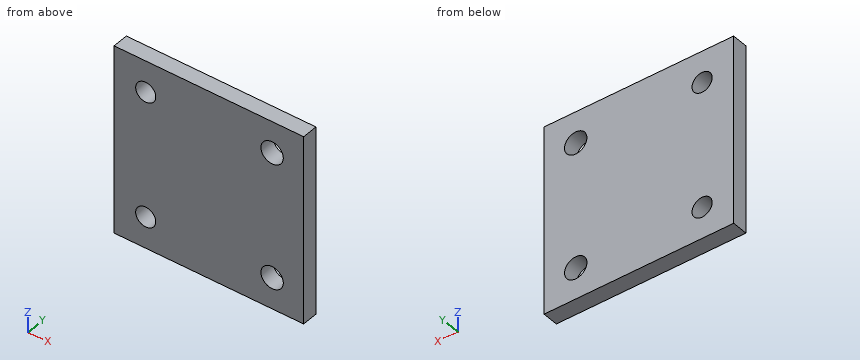
from build123d import *

# Parameters (mm, degrees)
SKETCH1_W              = 38.1
SKETCH1_H              = 38.1
BOSS_EXTRUDE1_DEPTH    = 1.5875
F_10_32_TAPPED_HOLE1_D = 4.0386
F_8_CLEARANCE_HOLE1_D  = 4.4958


with BuildPart() as part:
    # Sketch1 → Boss-Extrude1 (new, symmetric)
    with BuildSketch(Plane(origin=(0, 0, 0), x_dir=(1, 0, 0), z_dir=(0, 1, 0))):
        Rectangle(SKETCH1_W, SKETCH1_H)
    extrude(amount=BOSS_EXTRUDE1_DEPTH, both=True)

    # #10-32 Tapped Hole1 (through all)
    with Locations(Plane(origin=(0, 1.5875, 0), x_dir=(1, 0, 0), z_dir=(0, 1, 0))):
        with Locations((-12.7, 12.7), (-12.7, -12.7)):
            Hole(F_10_32_TAPPED_HOLE1_D / 2)

    # #8 Clearance Hole1 (through all)
    with Locations(Plane(origin=(0, 1.5875, 0), x_dir=(1, 0, 0), z_dir=(0, 1, 0))):
        with Locations((12.7, 12.7), (12.7, -12.7)):
            Hole(F_8_CLEARANCE_HOLE1_D / 2)


solid = part.part
Geometry: final body of the model. Coordinates: model frame, mm. Coordinates: 2 decimals unless noted, no trailing zeros. Order: outer loops, then holes, each group sorted by start corner. A loop starts at its lowest first (then second) coordinate and runs counter-clockwise, first axis right, second up. Notation, with made-up numbers: (23.5, -32) - (27.5, -32) arc R19 cw to (27.5, -20) - close; hole circle Ø9 at (13, -2). An arc over 180 degrees is marked (long way). Use one line per item in the form item = value.
1) Ray query, L1, parallel to X at y = 0.6, z = 12.7; L2, parallel to Z at x = -12.7, y = -0.7; L3, parallel to Z at x = 12.7, y = -0.5. Return the intervals inside material, ascending.
Solutions:
L1 = -19.05 to -14.72, -10.68 to 10.45, 14.95 to 19.05
L2 = -19.05 to -14.72, -10.68 to 10.68, 14.72 to 19.05
L3 = -19.05 to -14.95, -10.45 to 10.45, 14.95 to 19.05
2) Section C-C (y = 1.1). Return loops of the section in (x, z).
Solutions:
outline = (-19.05, -19.05) - (19.05, -19.05) - (19.05, 19.05) - (-19.05, 19.05) - close; hole circle Ø4.04 at (-12.7, -12.7); hole circle Ø4.04 at (-12.7, 12.7); hole circle Ø4.5 at (12.7, -12.7); hole circle Ø4.5 at (12.7, 12.7)
3) Section A-A (x = 12.7). Return loops of the section in (y, z), then the cut area to 3 significant figures.
Solutions:
outline = (-1.59, -19.05) - (1.59, -19.05) - (1.59, -14.95) - (-1.59, -14.95) - close; (-1.59, -10.45) - (1.59, -10.45) - (1.59, 10.45) - (-1.59, 10.45) - close; (-1.59, 14.95) - (1.59, 14.95) - (1.59, 19.05) - (-1.59, 19.05) - close
area = 92.4 mm^2
4) Section B-B (z = -12.7). Return loops of the section in (x, y).
Solutions:
outline = (-19.05, -1.59) - (-14.72, -1.59) - (-14.72, 1.59) - (-19.05, 1.59) - close; (-10.68, -1.59) - (10.45, -1.59) - (10.45, 1.59) - (-10.68, 1.59) - close; (14.95, -1.59) - (19.05, -1.59) - (19.05, 1.59) - (14.95, 1.59) - close
